Part model, mm, in its own coordinate system. A direction names the side the tool comes from. Coordinates: 2 decimals unless noted, no trailing zeros. Write each loop counter-clockwise with the first axis right and the second up, starting at its lowest first coordinate (ties: lowest second). Pieces come first, ordered by that corner, then holes. Notation, with made-up numbers: (42, 73) -> (64, 73) arc R25 cw to (64, 108) -> close; hole circle Ø8 at (-15.75, 51.5). An arc over 180 degrees is marked (long way). Write item = value, one per line.
from build123d import *

# Parameters (mm, degrees)
F0_W       = 12
F0_H       = 25
F0_W_2     = 25
F0_H_2     = 12
F1_DEPTH   = 5
F2_DEPTH   = 20
F3_R       = 10
F5_R       = 3.25
F6_DEPTH   = 25
F4_R       = 3
F4_R_2     = 3.25
F7_DEPTH   = 25
F8_SIZE2   = 11.99999
F8_SIZE    = 19.99999
F8_2_SIZE2 = 11.99999
F8_2_SIZE  = 19.99999
F9_SIZE    = 5


# Not quite as in the source:
# - a fillet or chamfer is up to 0.001 mm smaller than in the source, because OpenCascade refuses the exact size


with BuildPart() as f1:
    # F0 (on Top) → F1 (new body)
    with BuildSketch(Plane.XY):
        Polygon((0, 90), (0, 0), (90, 0), (90, 5), (60, 5), (35, 5), (5, 5), (5, 35), (5, 60), (5, 90), align=None)
        Polygon((90, 5), (5, 90), (5, 60), (17, 60), (17, 35), (5, 35), (5, 5), (35, 5), (35, 17), (60, 17), (60, 5), align=None)
        with Locations((11, 47.5)):
            Rectangle(F0_W, F0_H)
        with Locations((47.5, 11)):
            Rectangle(F0_W_2, F0_H_2)
    extrude(amount=F1_DEPTH)

    # F0 (on Top) → F2 (join)
    with BuildSketch(Plane.XY):
        Polygon((0, 90), (0, 0), (90, 0), (90, 5), (60, 5), (35, 5), (5, 5), (5, 35), (5, 60), (5, 90), align=None)
        with Locations((11, 47.5)):
            Rectangle(F0_W, F0_H)
        with Locations((47.5, 11)):
            Rectangle(F0_W_2, F0_H_2)
    extrude(amount=-F2_DEPTH)

    # F3
    f3_edges = [f1.edges().sort_by_distance(p)[0] for p in [
        (5, 5, -10),
        (2.5, 90, -20),
        (90, 2.5, -20),
    ]]
    fillet(f3_edges, radius=F3_R)

    # F5 (on face) → F6 (cut)
    with BuildSketch(Plane.XZ):
        with Locations((22.5, -10)):
            Circle(F5_R)
        with Locations((80, -10)):
            Circle(F5_R)
    extrude(amount=-F6_DEPTH, mode=Mode.SUBTRACT)

    # F4 (on face) → F7 (cut)
    with BuildSketch(Plane(origin=(0, 0, 0), x_dir=(0, -1, 0), z_dir=(-1, 0, 0))):
        with Locations((-22.5, -10)):
            Circle(F4_R)
        with Locations((-80, -10)):
            Circle(F4_R_2)
    extrude(amount=-F7_DEPTH, mode=Mode.SUBTRACT)

    # F8 (size 20 and 12 in the source; OpenCascade refuses exactly that, so slightly less here)
    f8_edges = [f1.edges().sort_by_distance(p)[0] for p in [
        (17, 47.5, -20),
    ]]
    f8_side = f1.faces().sort_by_distance((17, 47.5, -10))[0]
    chamfer(f8_edges, length=F8_SIZE, length2=F8_SIZE2, reference=f8_side)

    # F8#2 (size 20 and 12 in the source; OpenCascade refuses exactly that, so slightly less here)
    f8_2_edges = [f1.edges().sort_by_distance(p)[0] for p in [
        (47.5, 17, -20),
    ]]
    f8_2_side = f1.faces().sort_by_distance((47.5, 17, -10))[0]
    chamfer(f8_2_edges, length=F8_2_SIZE, length2=F8_2_SIZE2, reference=f8_2_side)

    # F9
    f9_edges = [f1.edges().sort_by_distance(p)[0] for p in [
        (0, 0, -7.5),
        (45, 0, 5),
        (0, 45, 5),
    ]]
    chamfer(f9_edges, length=F9_SIZE)


solid = f1.part
Q1. Saw through at B-B on y = 22.5. Give the cut face in (x, z), and give its area (3 significant figures).
Model answer:
outline = (0, -20) -> (5, -20) -> (5, -13) -> (0, -13) -> close; (0, -7) -> (5, -7) -> (5, 0) -> (72.5, 0) -> (72.5, 5) -> (5, 5) -> (0, 0) -> close
area = 420 mm²
Q2. Mould opens along Y. For faces 5 (the face through (90, 2, -4)), 6 (the face through (10, 60, -8)), 7 (the face through (2.5, 25.5, -9.9)), 8 (the face through (47, 3, 3)) say: released by +Y, released by -Y, zero draft, split by the parting line, or undercut.
Model answer:
face_5 = zero draft
face_6 = released by +Y
face_7 = undercut
face_8 = released by -Y
Q3. Saw through at A-A on x = 22.5. Give the cut face in (y, z).
Model answer:
outline = (0, -20) -> (5, -20) -> (5, -13.25) -> (0, -13.25) -> close; (0, -6.75) -> (5, -6.75) -> (5, 0) -> (72.5, 0) -> (72.5, 5) -> (5, 5) -> (0, 0) -> close
Q4. Probe line 1 (Z direction, x = 80, y = 2); line 2 (Y direction, x = 65, z = -17.25). List the from-to ranges inside material, lowest first. Write a range as from..to.
Model answer:
line_1 = -20..-13.25, -6.75..2
line_2 = 0..5
Q5. Which spindle directions (+Z, -Z, +X, -X, +Y, -Y) get a long thin tool onto all of the face, cutting with end or side? Do faces 1 (the face through (7.85, 8.01, -10.14)), 2 (the face through (3.5, 3.4, 1.9)), 3 (the face through (60, 10, -8)), 4 (the face through (10, 35, -8)). Say none if no direction does.
Model answer:
face_1 = -Z
face_2 = +Z, -X, -Y
face_3 = -Z, +X, +Y
face_4 = -Z, +X
Q6. Saw through at D-D on z = -8.75. Count the separate pieces of the cut face and the enclosed holes in it, and give its area (3 significant figures).
Model answer:
separate_pieces = 5
enclosed_holes = 0
area = 1,100 mm²
Q7. Pin check, flat tips, straight feed: pin 1 (8.5 mm diameter, centred on y = 80, z = -10, fed in from +X); pin 2 (8.5 mm diameter, centred on x = 80, z = -10, fed in from +Y); pin 3 (6 mm diameter, centred on y = 13.5, z = -11, fed in from +X); pin 4 (6 mm diameter, centred on x = 43.5, z = -15.5, fed in from -Y). Stop position of each tip, or through.
Model answer:
pin_1 = 5
pin_2 = 5
pin_3 = 60
pin_4 = 0
Q8. Saw through at C-C on y = 64.5. Give the cut face in (x, z), and give its area (3 significant figures).
Model answer:
outline = (0, -20) -> (5, -20) -> (5, 0) -> (30.5, 0) -> (30.5, 5) -> (5, 5) -> (0, 0) -> close
area = 240 mm²
